Can you work these out from the model? Positions are in its coordinate system, mm. A direction names the side the tool comes from. Give positions to 0.01 mm unless a question says otherwise; leave off trailing zeros. Loops run counter-clockwise (first coordinate to the right, second up) from the corner with the lowest first, then second, coordinate; pieces in that order, holes last.
from build123d import *

# Parameters (mm, degrees)
F0_R     = 8.5
F1_DEPTH = 4
F2_R     = 5
F3_DEPTH = 100
F7_DEPTH = 5
F8_R     = 0.5
F9_DEPTH = 120


with BuildPart() as f1:
    # F0 (on Top) → F1 (new body)
    with BuildSketch(Plane.XY):
        Circle(F0_R)
    extrude(amount=F1_DEPTH)

    # F2 (on Top) → F3 (join)
    with BuildSketch(Plane.XY):
        Circle(F2_R)
    extrude(amount=F3_DEPTH)

    # F4 (on Right) → F5 (revolve)
    with BuildSketch(Plane.YZ):
        Polygon((3, 105), (0, 105), (0, 100), (4, 100), align=None)
    revolve(axis=Axis((0, 0, 102.5), (0, 0, -1)))

    # F6 (on face) → F7 (join)
    with BuildSketch(Plane.XY.offset(105)):
        Polygon((0.866025, -0.5), (0.866025, 0.5), (0, 1), (-0.866025, 0.5), (-0.866025, -0.5), (0, -1), align=None)
    extrude(amount=F7_DEPTH)

    # F8 (on face) → F9 (cut)
    with BuildSketch(Plane.XY.offset(110)):
        Circle(F8_R)
    extrude(amount=-F9_DEPTH, mode=Mode.SUBTRACT)


solid = f1.part
(1) Which directions (+Z, -Z, +X, -X, +Y, -Y) give clear straight access to the entire face, cutting with the end or side of a thin tool? Please do faces 1 (the flat face through (4, -4, 4)), 2 (the cylindrical face through (4.57, 7.167, 1.972)).
Returned:
face 1: +Z
face 2: +Z, -Z
(2) Suppose I cut it at B-B on x = -7. List the corners of the cut face in (y, z) for me.
Returned:
outline: (-4.82, 0) - (4.82, 0) - (4.82, 4) - (-4.82, 4) - close
(3) Will these pins go through, and if not, where does the flat tip stop? P1, Ø1.1, axis at y = 0, z = 108.5, coming from the -X side; P2, Ø8, axis at x = -1.5, z = 81, coming from the -Y side; P3, Ø10, axis at y = 0.5, z = 79, coming from the +X side.
Returned:
P1: stops at x = -0.87
P2: stops at y = -5
P3: stops at x = 5
(4) Please list where these lines run through material, in increasing order: probe 1 along Y at (x, z) = (0, 62.5); probe 2 along Z at (x, y) = (-2, 5); probe 3 along Y at (x, z) = (4, 36.5).
Returned:
probe 1: y = -5 to -0.5, 0.5 to 5
probe 2: z = 0 to 4
probe 3: y = -3 to 3
(5) Suppose I cut it at A-A on z = 87.5. List the corners of the cut face in (x, y) for me.
Returned:
outline: circle Ø10 at (0, 0); hole circle Ø1 at (0, 0)
